The listing builds one solid part. Answer for the finished solid, in the listing's coordinates (mm). Coordinates: 2 decimals unless noted, no trailing zeros. Order: outer loops, then holes, each group sorted by start corner. A loop starts at its lowest first (then second) coordinate and runs counter-clockwise, first axis right, second up. Notation, with made-up numbers: (81.5, 87.5) -> (108.5, 87.5) arc R25 cw to (108.5, 101.5) -> close; hole circle Ø6 at (59.5, -36.5). An arc over 180 degrees is marked (long way). Return JSON: item names as keys, results as strings.
```python
from build123d import *

# Parameters (mm, degrees)
SKETCH5_R          = 0.5
CUT_EXTRUDE1_DEPTH = 21.615528128
CIRPATTERN1_COUNT  = 4
SKETCH6_R          = 0.5
CUT_EXTRUDE2_DEPTH = 21.615528225


with BuildPart() as part:
    # Sketch1 → Revolve2 (revolve)
    with BuildSketch(Plane.XY):
        with BuildLine():
            Line((10, 5), (10, 0))
            Line((10, 0), (9.5, 0))
            Line((9.5, 0), (9.5, 5))
            ThreePointArc((9.5, 5), (6.717514421, 11.717514421), (0, 14.5))
            Line((0, 14.5), (0, 15))
            ThreePointArc((0, 15), (7.071067812, 12.071067812), (10, 5))
        make_face()
    revolve(axis=Axis((0, 0, 0), (0, 1, 0)))

    # Sketch5 → Cut-Extrude1 (cut, through all)
    with BuildSketch(Plane.XY):
        with Locations(Location((0, 5, 0), (0, 0, 180))):
            Circle(SKETCH5_R)
    cut_extrude1 = extrude(amount=CUT_EXTRUDE1_DEPTH, mode=Mode.SUBTRACT)

    # CirPattern1: Cut-Extrude1 ×4 about axis
    cirpattern1_axis = Axis((0, 0, 0), (0, -1, 0))
    for i in range(1, CIRPATTERN1_COUNT):
        add(cut_extrude1.rotate(cirpattern1_axis, i * 360 / CIRPATTERN1_COUNT), mode=Mode.SUBTRACT)

    # Sketch6 → Cut-Extrude2 (cut, through all)
    with BuildSketch(Plane(origin=(0, 0, 0), x_dir=(1, 0, 0), z_dir=(0, 1, 0))):
        with Locations(Location((0, 0, 0), (0, 0, 90))):
            Circle(SKETCH6_R)
    extrude(amount=CUT_EXTRUDE2_DEPTH, mode=Mode.SUBTRACT)


solid = part.part
```
Item 1: The part is cut by section B-B on x = 0. Determine the outline of the cut face in (y, z), plus the area to 3 significant figures.
Answer list:
{"outline": "(0, -10) -> (4.5, -10) -> (4.5, -9.5) -> (0, -9.5) -> close; (0, 9.5) -> (4.5, 9.5) -> (4.5, 10) -> (0, 10) -> close; (5.5, -9.99) arc R10 ccw to (14.99, -0.5) -> (14.49, -0.5) arc R9.5 cw to (5.5, -9.49) -> close; (5.5, 9.49) arc R9.5 cw to (14.49, 0.5) -> (14.99, 0.5) arc R10 ccw to (5.5, 9.99) -> close", "area": "18.8 mm2"}
Item 2: Determine the mould class of faces 1 (the cylindrical face through (8.776, 2.535, 3.639)), 2 (the cylindrical face through (-0.065, 4.504, -9.74)), 3 (the cylindrical face through (-2.17, 2.47, 9.76)) for opening direction Z: pulls with the +Z half, pulls with the -Z half, needs draft (parallel to the pull), parting line crosses it, or undercut.
Answer list:
{"face 1": "undercut", "face 2": "needs draft", "face 3": "parting line crosses it"}
Item 3: The part is cut by section D-D on z = 5.25. Determine the outline of the cut face in (x, y).
Answer list:
{"outline": "(-8.51, 0) -> (-7.92, 0) -> (-7.92, 5) arc R7.92 cw to (7.92, 5) -> (7.92, 0) -> (8.51, 0) -> (8.51, 5) arc R8.51 ccw to (-8.51, 5) -> close"}
Item 4: The part is cut by section C-C on x = -8. Determine the outline of the cut face in (y, z).
Answer list:
{"outline": "(0, -6) -> (5, -6) arc R6 ccw to (5, 6) -> (0, 6) -> (0, 5.12) -> (5, 5.12) arc R5.12 cw to (5, -5.12) -> (0, -5.12) -> close"}
Item 5: Flat-ended cylindrical pins translate along their axes: pin 1 (2 mm diameter, centred on x = -5.5, y = 12, fed in from +Z); pin 2 (1 mm diameter, centred on x = 3.5, y = 11.5, fed in from +Z); pin 3 (1.5 mm diameter, centred on x = 0, y = 5.5, fed in from +Z). Find the tip coordinate at first contact, or state that the pin passes through.
Answer list:
{"pin 1": "z = 6.13", "pin 2": "z = 7.25", "pin 3": "z = 9.99"}
Item 6: The part is cut by section A-A on z = 0. Determine the outline of the cut face in (x, y), plus the area to 3 significant figures.
Answer list:
{"outline": "(-10, 0) -> (-9.5, 0) -> (-9.5, 4.5) -> (-10, 4.5) -> close; (-9.99, 5.5) -> (-9.49, 5.5) arc R9.5 cw to (-0.5, 14.49) -> (-0.5, 14.99) arc R10 ccw to start; (0.5, 14.49) arc R9.5 cw to (9.49, 5.5) -> (9.99, 5.5) arc R10 ccw to (0.5, 14.99) -> close; (9.5, 0) -> (10, 0) -> (10, 4.5) -> (9.5, 4.5) -> close", "area": "18.8 mm2"}
Item 7: Find the intervals of material crossed by probe 1 along Z at (x, y) = (1.5, 9.75); probe 2 along Z at (x, y) = (-0.5, 5.25); probe 3 along X at (y, z) = (4, 4), in increasing order.
Answer list:
{"probe 1": "-8.67 to -8.09, 8.09 to 8.67", "probe 2": "-9.98 to -9.48, 9.48 to 9.98", "probe 3": "-9.17 to -8.62, 8.62 to 9.17"}
